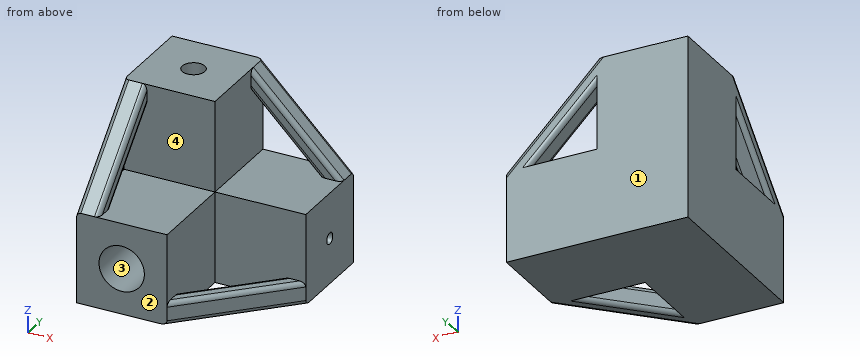
from build123d import *

# Parameters (mm, degrees)
F0_W          = 25.4
F0_H          = 25.4
F1_DEPTH      = 12.7
F2_R          = 3.175
F3_DEPTH      = 5.08
F4_R          = 1.5875
F5_DEPTH      = 5.08
F6_R          = 6.35
F7_DEPTH      = 12.7
F8_SIZE       = 1.27
F9_SIZE       = 0.396875
F10_SIZE      = 0.79375
F11_W         = 25.4
F11_H         = 25.4
F11_R         = 1.5875
F12_DEPTH     = 25.4
F13_W         = 25.4
F13_H         = 25.4
F13_R         = 6.35
F14_DEPTH     = 25.4
F15_W         = 25.4
F15_H         = 25.4
F15_R         = 3.175
F16_DEPTH     = 25.4
F18_DEPTH     = 6.35
F20_DEPTH     = 6.35
F22_DEPTH     = 6.35
F23_T1_DEPTH  = 42.2710244843
F23_T3_DEPTH  = 42.2710244843
F23_T5_DEPTH  = 42.2710244843
F23_T10_DEPTH = 42.2710244843
F23_T16_DEPTH = 33.2907683632
F23_T22_DEPTH = 33.2907683632
F23_T28_DEPTH = 42.2710244843
F23_T34_DEPTH = 33.2907683632
F23_T40_DEPTH = 33.2907683632
F23_T46_DEPTH = 42.2710244843
F23_T52_DEPTH = 33.2907683632
F23_T58_DEPTH = 33.2907683632


# Not quite as in the source:
# - a fillet or chamfer that OpenCascade refuses, or shapes differently, is made with other operations: its cross-section is extruded or revolved along the edge and cut away or added


with BuildPart() as f1:
    # F0 (on Top) → F1 (new body, symmetric)
    with BuildSketch(Plane.XY):
        Rectangle(F0_W, F0_H)
    extrude(amount=F1_DEPTH, both=True)

    # F2 (on face) → F3 (cut)
    with BuildSketch(Plane.XY.offset(12.7)):
        Circle(F2_R)
    extrude(amount=-F3_DEPTH, mode=Mode.SUBTRACT)

    # F4 (on face) → F5 (cut)
    with BuildSketch(Plane.YZ.offset(12.7)):
        Circle(F4_R)
    extrude(amount=-F5_DEPTH, mode=Mode.SUBTRACT)

    # F6 (on face) → F7 (cut)
    with BuildSketch(Plane.XZ.offset(12.7)):
        Circle(F6_R)
    extrude(amount=-F7_DEPTH, mode=Mode.SUBTRACT)

    # F8
    f8_edges = [f1.edges().sort_by_distance(p)[0] for p in [
        (-6.35, 0, 0),
    ]]
    chamfer(f8_edges, length=F8_SIZE)

    # F9
    f9_edges = [f1.edges().sort_by_distance(p)[0] for p in [
        (7.62, -1.5875, 0),
    ]]
    chamfer(f9_edges, length=F9_SIZE)

    # F10
    f10_edges = [f1.edges().sort_by_distance(p)[0] for p in [
        (-3.175, 0, 7.62),
    ]]
    chamfer(f10_edges, length=F10_SIZE)

    # F11 (on face) → F12 (join)
    with BuildSketch(Plane.YZ.offset(12.7)):
        Rectangle(F11_W, F11_H)
        Circle(F11_R, mode=Mode.SUBTRACT)
    extrude(amount=F12_DEPTH)

    # F13 (on face) → F14 (join)
    with BuildSketch(Plane.XZ.offset(12.7)):
        Rectangle(F13_W, F13_H)
        Circle(F13_R, mode=Mode.SUBTRACT)
    extrude(amount=F14_DEPTH)

    # F15 (on face) → F16 (join)
    with BuildSketch(Plane.XY.offset(12.7)):
        Rectangle(F15_W, F15_H)
        Circle(F15_R, mode=Mode.SUBTRACT)
    extrude(amount=F16_DEPTH)

    # F17 (on face) → F18 (join)
    with BuildSketch(Plane(origin=(0, 0, -12.7), x_dir=(1, 0, 0), z_dir=(0, 0, -1))):
        Polygon((38.1, 12.7), (12.7, 38.1), (12.7, 31.75), (31.75, 12.7), align=None)
    extrude(amount=-F18_DEPTH)

    # F19 (on face) → F20 (join)
    with BuildSketch(Plane(origin=(0, 12.7, 0), x_dir=(-1, 0, 0), z_dir=(0, 1, 0))):
        Polygon((-12.7, 38.1), (-38.1, 12.7), (-31.75, 12.7), (-12.7, 31.75), align=None)
    extrude(amount=-F20_DEPTH)

    # F21 (on face) → F22 (join)
    with BuildSketch(Plane(origin=(-12.7, 0, 0), x_dir=(0, -1, 0), z_dir=(-1, 0, 0))):
        Polygon((38.1, 12.7), (12.7, 38.1), (12.7, 31.75), (31.75, 12.7), align=None)
    extrude(amount=-F22_DEPTH)

    # F23: fillet of radius 1.27 on 12 edges, made by hand

    # F23_s2 → F23_t1 (cut)
    with BuildSketch(Plane(origin=(-14.9450640303, 0, 14.9450640303), x_dir=(0, 1, 0), z_dir=(0.7071067812, 0, -0.7071067812))):
        with BuildLine():
            ThreePointArc((11.43, 35.9210244843), (12.3280256121, 35.5490500964), (12.7, 34.6510244843))
            Line((12.7, 34.6510244843), (12.7, 35.9210244843))
            Line((12.7, 35.9210244843), (11.43, 35.9210244843))
        make_face()
    extrude(amount=F23_T1_DEPTH, mode=Mode.SUBTRACT)

    # F23_s4 → F23_t3 (cut)
    with BuildSketch(Plane(origin=(0, -14.9450640303, -14.9450640303), x_dir=(1, 0, 0), z_dir=(0, 0.7071067812, 0.7071067812))):
        with BuildLine():
            ThreePointArc((-11.43, -35.9210244843), (-12.3280256121, -35.5490500964), (-12.7, -34.6510244843))
            Line((-12.7, -34.6510244843), (-12.7, -35.9210244843))
            Line((-12.7, -35.9210244843), (-11.43, -35.9210244843))
        make_face()
    extrude(amount=F23_T3_DEPTH, mode=Mode.SUBTRACT)

    # F23_s6 → F23_t5 (cut)
    with BuildSketch(Plane(origin=(14.9450640303, 14.9450640303, 0), x_dir=(0, 0, 1), z_dir=(-0.7071067812, -0.7071067812, 0))):
        with BuildLine():
            ThreePointArc((-11.43, -35.9210244843), (-12.3280256121, -35.5490500964), (-12.7, -34.6510244843))
            Line((-12.7, -34.6510244843), (-12.7, -35.9210244843))
            Line((-12.7, -35.9210244843), (-11.43, -35.9210244843))
        make_face()
    extrude(amount=F23_T5_DEPTH, mode=Mode.SUBTRACT)


with BuildPart() as f23_tool8:
    # F23_s9 → F23_t10 (new body)
    with BuildSketch(Plane(origin=(-14.9450640303, 0, 14.9450640303), x_dir=(0, 1, 0), z_dir=(0.7071067812, 0, -0.7071067812))):
        with BuildLine():
            ThreePointArc((7.62, 35.9210244843), (6.7219743879, 35.5490500964), (6.35, 34.6510244843))
            Line((6.35, 34.6510244843), (6.35, 35.9210244843))
            Line((6.35, 35.9210244843), (7.62, 35.9210244843))
        make_face()
    extrude(amount=F23_T10_DEPTH)

    split(bisect_by=Plane.YZ.offset(12.7), keep=Keep.TOP)

    split(bisect_by=Plane.XY.offset(12.7), keep=Keep.TOP)


with BuildPart() as f1_1:
    add(f1.part)

    # F23_t7: cut F23_tool8
    add(f23_tool8.part, mode=Mode.SUBTRACT)


with BuildPart() as f23_tool14:
    # F23_s15 → F23_t16 (new body)
    with BuildSketch(Plane(origin=(11.7700640303, 0, -11.7700640303), x_dir=(0, 1, 0), z_dir=(-0.7071067812, 0, 0.7071067812))):
        with BuildLine():
            ThreePointArc((12.7, -32.7008964237), (12.3280256121, -31.8028708116), (11.43, -31.4308964237))
            Line((11.43, -31.4308964237), (12.7, -31.4308964237))
            Line((12.7, -31.4308964237), (12.7, -32.7008964237))
        make_face()
    extrude(amount=F23_T16_DEPTH)

    split(bisect_by=Plane.YZ.offset(12.7), keep=Keep.TOP)

    split(bisect_by=Plane.XY.offset(12.7), keep=Keep.TOP)


with BuildPart() as f1_2:
    add(f1_1.part)

    # F23_t13: cut F23_tool14
    add(f23_tool14.part, mode=Mode.SUBTRACT)


with BuildPart() as f23_tool20:
    # F23_s21 → F23_t22 (new body)
    with BuildSketch(Plane(origin=(11.7700640303, 0, -11.7700640303), x_dir=(0, 1, 0), z_dir=(-0.7071067812, 0, 0.7071067812))):
        with BuildLine():
            ThreePointArc((7.62, -31.4308964237), (6.7219743879, -31.8028708116), (6.35, -32.7008964237))
            Line((6.35, -32.7008964237), (6.35, -31.4308964237))
            Line((6.35, -31.4308964237), (7.62, -31.4308964237))
        make_face()
    extrude(amount=F23_T22_DEPTH)

    split(bisect_by=Plane.YZ.offset(12.7), keep=Keep.TOP)

    split(bisect_by=Plane.XY.offset(12.7), keep=Keep.TOP)


with BuildPart() as f1_3:
    add(f1_2.part)

    # F23_t19: cut F23_tool20
    add(f23_tool20.part, mode=Mode.SUBTRACT)


with BuildPart() as f23_tool26:
    # F23_s27 → F23_t28 (new body)
    with BuildSketch(Plane(origin=(0, -14.9450640303, -14.9450640303), x_dir=(1, 0, 0), z_dir=(0, 0.7071067812, 0.7071067812))):
        with BuildLine():
            ThreePointArc((-7.62, -35.9210244843), (-6.7219743879, -35.5490500964), (-6.35, -34.6510244843))
            Line((-6.35, -34.6510244843), (-6.35, -35.9210244843))
            Line((-6.35, -35.9210244843), (-7.62, -35.9210244843))
        make_face()
    extrude(amount=F23_T28_DEPTH)

    split(bisect_by=Plane.XZ.offset(12.7), keep=Keep.TOP)

    split(bisect_by=Plane.XY.offset(12.7), keep=Keep.TOP)


with BuildPart() as f1_4:
    add(f1_3.part)

    # F23_t25: cut F23_tool26
    add(f23_tool26.part, mode=Mode.SUBTRACT)


with BuildPart() as f23_tool32:
    # F23_s33 → F23_t34 (new body)
    with BuildSketch(Plane(origin=(0, 11.7700640303, 11.7700640303), x_dir=(1, 0, 0), z_dir=(0, -0.7071067812, -0.7071067812))):
        with BuildLine():
            ThreePointArc((-6.35, 32.7008964237), (-6.7219743879, 31.8028708116), (-7.62, 31.4308964237))
            Line((-7.62, 31.4308964237), (-6.35, 31.4308964237))
            Line((-6.35, 31.4308964237), (-6.35, 32.7008964237))
        make_face()
    extrude(amount=F23_T34_DEPTH)

    split(bisect_by=Plane.XZ.offset(12.7), keep=Keep.TOP)

    split(bisect_by=Plane.XY.offset(12.7), keep=Keep.TOP)


with BuildPart() as f1_5:
    add(f1_4.part)

    # F23_t31: cut F23_tool32
    add(f23_tool32.part, mode=Mode.SUBTRACT)


with BuildPart() as f23_tool38:
    # F23_s39 → F23_t40 (new body)
    with BuildSketch(Plane(origin=(0, 11.7700640303, 11.7700640303), x_dir=(1, 0, 0), z_dir=(0, -0.7071067812, -0.7071067812))):
        with BuildLine():
            ThreePointArc((-12.7, 32.7008964237), (-12.3280256121, 31.8028708116), (-11.43, 31.4308964237))
            Line((-11.43, 31.4308964237), (-12.7, 31.4308964237))
            Line((-12.7, 31.4308964237), (-12.7, 32.7008964237))
        make_face()
    extrude(amount=F23_T40_DEPTH)

    split(bisect_by=Plane.XZ.offset(12.7), keep=Keep.TOP)

    split(bisect_by=Plane.XY.offset(12.7), keep=Keep.TOP)


with BuildPart() as f1_6:
    add(f1_5.part)

    # F23_t37: cut F23_tool38
    add(f23_tool38.part, mode=Mode.SUBTRACT)


with BuildPart() as f23_tool44:
    # F23_s45 → F23_t46 (new body)
    with BuildSketch(Plane(origin=(14.9450640303, 14.9450640303, 0), x_dir=(0, 0, 1), z_dir=(-0.7071067812, -0.7071067812, 0))):
        with BuildLine():
            ThreePointArc((-7.62, -35.9210244843), (-6.7219743879, -35.5490500964), (-6.35, -34.6510244843))
            Line((-6.35, -34.6510244843), (-6.35, -35.9210244843))
            Line((-6.35, -35.9210244843), (-7.62, -35.9210244843))
        make_face()
    extrude(amount=F23_T46_DEPTH)

    split(bisect_by=Plane.YZ.offset(12.7), keep=Keep.TOP)

    split(bisect_by=Plane.XZ.offset(12.7), keep=Keep.TOP)


with BuildPart() as f1_7:
    add(f1_6.part)

    # F23_t43: cut F23_tool44
    add(f23_tool44.part, mode=Mode.SUBTRACT)


with BuildPart() as f23_tool50:
    # F23_s51 → F23_t52 (new body)
    with BuildSketch(Plane(origin=(-11.7700640303, -11.7700640303, 0), x_dir=(0, 0, 1), z_dir=(0.7071067812, 0.7071067812, 0))):
        with BuildLine():
            ThreePointArc((-12.7, 32.7008964237), (-12.3280256121, 31.8028708116), (-11.43, 31.4308964237))
            Line((-11.43, 31.4308964237), (-12.7, 31.4308964237))
            Line((-12.7, 31.4308964237), (-12.7, 32.7008964237))
        make_face()
    extrude(amount=F23_T52_DEPTH)

    split(bisect_by=Plane.YZ.offset(12.7), keep=Keep.TOP)

    split(bisect_by=Plane.XZ.offset(12.7), keep=Keep.TOP)


with BuildPart() as f1_8:
    add(f1_7.part)

    # F23_t49: cut F23_tool50
    add(f23_tool50.part, mode=Mode.SUBTRACT)


with BuildPart() as f23_tool56:
    # F23_s57 → F23_t58 (new body)
    with BuildSketch(Plane(origin=(-11.7700640303, -11.7700640303, 0), x_dir=(0, 0, 1), z_dir=(0.7071067812, 0.7071067812, 0))):
        with BuildLine():
            ThreePointArc((-6.35, 32.7008964237), (-6.7219743879, 31.8028708116), (-7.62, 31.4308964237))
            Line((-7.62, 31.4308964237), (-6.35, 31.4308964237))
            Line((-6.35, 31.4308964237), (-6.35, 32.7008964237))
        make_face()
    extrude(amount=F23_T58_DEPTH)

    split(bisect_by=Plane.YZ.offset(12.7), keep=Keep.TOP)

    split(bisect_by=Plane.XZ.offset(12.7), keep=Keep.TOP)


with BuildPart() as f1_9:
    add(f1_8.part)

    # F23_t55: cut F23_tool56
    add(f23_tool56.part, mode=Mode.SUBTRACT)


solid = f1_9.part
Can you work these out from the model? Positions are in its coordinate system, mm. Face numbers are marked on the shaded views. Coordinates: 2 decimals unless noted, no trailing zeros. Loops run counter-clockwise (first coordinate to the right, second up) from the corner with the lowest first, then second, coordinate; pieces in that order, holes last. Notation, with made-up numbers: (-9, 25.5) - (28, 25.5) arc R9 ccw to (28, 31.5) - close; hole circle Ø1 at (36.25, 81). An arc over 180 degrees is marked (long way). Put each result on its own line as item: value. Start each with the question number.
Item 1: Suppose I cut it at B-B (x = 0). Please give me the cut outline in (y, z) (3 decimals).
Item 2: If I drill on line 1 along Y through (x, z) = (0, 18.25) (3 decimals); line 2 along Z through (x, y) = (0, -23); line 3 along Z through (x, y) = (22.5, 0), over which ranges is the centre line in solid material (lowest first)?
Item 3: For pin 1 (7.5 mm diameter, centred on y = 1.5, z = 26.5, fed in from +X); pin 2 (16.5 mm diameter, centred on x = 0, z = 0, fed in from -Y); pin 3 (10 mm diameter, centred on x = 23.5, y = -16, fed in from +Z); pin 4 (4 mm diameter, centred on x = 0, y = 0, fed in from +Z), each with a flat end and sliding along its axis, tell me the tip position at first contact or that it passes through.
Item 4: Suppose I cut it at A-A (z = -8.5). Please give me the cut outline in (x, y), and give its area (3 significant figures).
Item 5: Suppose I cut it at C-C (x = 9). Please give me the cut outline in (y, z) (1 decimal), and give its area (3 significant figures).
Item 6: Suppose I cut it at D-D (z = 0). Please give me the cut outline in (x, y).
Item 7: If we mould it in two halves opening along Y, with no side actions, what happens to the marked faces 1, 2, 3 and 4? For each: +Y half, -Y half, draft (parallel to the pull), parting line (faces both ways), or undercut.
Here are the results:
1. outline: (-38.1, -12.7) - (12.7, -12.7) - (12.7, 38.1) - (3.175, 38.1) - (3.175, 8.414) - (2.381, 7.62) - (-2.381, 7.62) - (-3.175, 8.414) - (-3.175, 38.1) - (-12.7, 38.1) - (-12.7, 12.7) - (-38.1, 12.7) - (-38.1, 6.35) - (-1.27, 6.35) - (0, 5.08) - (0, -5.08) - (-1.27, -6.35) - (-38.1, -6.35) - close
2. line 1: -12.7 to -3.175, 3.175 to 12.7
2. line 2: -12.7 to -6.35, 6.35 to 12.7
2. line 3: -12.7 to -1.59, 1.59 to 12.7
3. pin 1: x = 12.7
3. pin 2: y = -38.1
3. pin 3: z = 12.7
3. pin 4: z = 7.62
4. outline: (-12.7, -38.1) - (12.7, -38.1) - (38.1, -12.7) - (38.1, 12.7) - (-12.7, 12.7) - close; hole (12.7, -31.75) - (31.75, -12.7) - (12.7, -12.7) - close
4. area: 2,080 mm²
5. outline: (-38.1, -12.7) - (12.7, -12.7) - (12.7, 38.1) - (-12.7, 38.1) - (-12.7, 12.7) - (-38.1, 12.7) - close; hole circle Ø3.2 at (0, 0)
5. area: 1,930 mm²
6. outline: (-12.7, -38.1) - (-6.35, -38.1) - (-6.35, -1.27) - (-5.08, 0) - (5.08, 0) - (6.35, -1.27) - (6.35, -38.1) - (12.7, -38.1) - (12.7, -12.7) - (38.1, -12.7) - (38.1, -1.59) - (8.02, -1.59) - (7.62, -1.19) - (7.62, 1.19) - (8.02, 1.59) - (38.1, 1.59) - (38.1, 12.7) - (-12.7, 12.7) - close
7. face 1: +Y half
7. face 2: -Y half
7. face 3: draft
7. face 4: undercut
